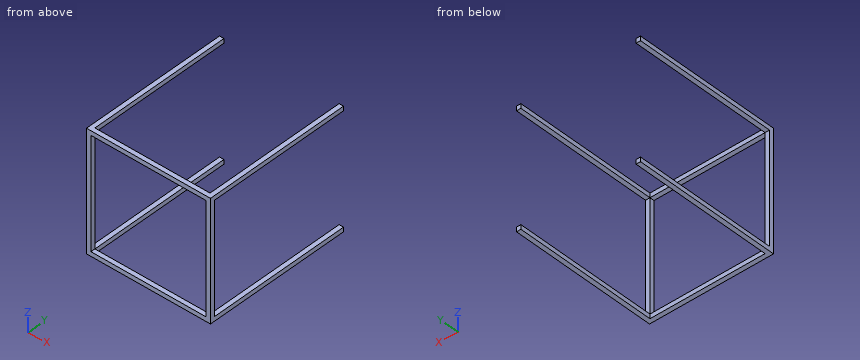
```python
from build123d import *

# Parameters (mm, degrees)
SKETCH1_W           = 1320.8
SKETCH1_H           = 50.8
SKETCH1_W_2         = 50.8
SKETCH1_H_2         = 1270
BOSS_EXTRUDE1_DEPTH = 50.8
SKETCH1_3_W         = 50.8
SKETCH1_3_H         = 50.8
BOSS_EXTRUDE2_DEPTH = 1689.1


with BuildPart() as part:
    # Sketch1 → Boss-Extrude1 (new body)
    with BuildSketch(Plane(origin=(0, 0, 0), x_dir=(1, 0, 0), z_dir=(0, 1, 0))):
        with Locations((0, 660.4)):
            Rectangle(SKETCH1_W, SKETCH1_H)
        with Locations((-685.8, 0)):
            Rectangle(SKETCH1_W_2, SKETCH1_H_2)
        with Locations((-685.8, 660.4)):
            Rectangle(SKETCH1_W_2, SKETCH1_H)
        with Locations((-685.8, -660.4)):
            Rectangle(SKETCH1_W_2, SKETCH1_H)
        with Locations((0, -660.4)):
            Rectangle(SKETCH1_W, SKETCH1_H)
        with Locations((685.8, -660.4)):
            Rectangle(SKETCH1_W_2, SKETCH1_H)
        with Locations((685.8, 0)):
            Rectangle(SKETCH1_W_2, SKETCH1_H_2)
        with Locations((685.8, 660.4)):
            Rectangle(SKETCH1_W_2, SKETCH1_H)
    extrude(amount=BOSS_EXTRUDE1_DEPTH)

    # Sketch1<3> → Boss-Extrude2 (add)
    with BuildSketch(Plane(origin=(0, 0, 0), x_dir=(1, 0, 0), z_dir=(0, 1, 0))):
        with Locations((-685.8, -660.4)):
            Rectangle(SKETCH1_3_W, SKETCH1_3_H)
        with Locations((-685.8, 660.4)):
            Rectangle(SKETCH1_3_W, SKETCH1_3_H)
        with Locations((685.8, 660.4)):
            Rectangle(SKETCH1_3_W, SKETCH1_3_H)
        with Locations((685.8, -660.4)):
            Rectangle(SKETCH1_3_W, SKETCH1_3_H)
    extrude(amount=BOSS_EXTRUDE2_DEPTH)


solid = part.part
```
Here's how the part is built. I have some questions about the finished solid (model axes, mm). Round coordinates to 2 decimals unless told otherwise and drop trailing zeros. Write each loop counter-clockwise with the first axis right and the second up, starting at its lowest first coordinate (ties: lowest second). Pieces come first, ordered by that corner, then holes.
Q1. If we section it at B-B on z = -70.5: Write out the boundary of the cut face in (x, y), plus the area to 3 significant figures.
Q2. If we section it at A-A on y = 1107.5: Write out the boundary of the cut face in (x, z), plus the area to 3 significant figures.
Q3. Will this pin go through, and if not, where does the flat tip stop? P1, Ø15, axis at x = -686.5, z = -62, coming from the +Y side.
Q4. If we section it at C-C on x = 53.5: Write out the boundary of the cut face in (y, z).
Answer below:
1. outline: (-711.2, 0) - (-660.4, 0) - (-660.4, 50.8) - (-711.2, 50.8) - close; (660.4, 0) - (711.2, 0) - (711.2, 50.8) - (660.4, 50.8) - close
1. area: 5,160 mm2
2. outline: (-711.2, -685.8) - (-660.4, -685.8) - (-660.4, -635) - (-711.2, -635) - close; (-711.2, 635) - (-660.4, 635) - (-660.4, 685.8) - (-711.2, 685.8) - close; (660.4, -685.8) - (711.2, -685.8) - (711.2, -635) - (660.4, -635) - close; (660.4, 635) - (711.2, 635) - (711.2, 685.8) - (660.4, 685.8) - close
2. area: 10,300 mm2
3. P1: stops at y = 50.8
4. outline: (0, -685.8) - (50.8, -685.8) - (50.8, -635) - (0, -635) - close; (0, 635) - (50.8, 635) - (50.8, 685.8) - (0, 685.8) - close
